from build123d import *

# Parameters (mm, degrees)
SKETCH1_W            = 20
SKETCH1_H            = 20
BOSS_EXTRUDE1_DEPTH  = 7.5
SKETCH1_3_W          = 20
SKETCH1_3_H          = 20
CUT_EXTRUDE2_DEPTH   = 1.5
SKETCH3_W            = 10
SKETCH3_H            = 20
BOSS_EXTRUDE2_DEPTH  = 1.5
MOUNTHOLE_DEPTH      = 17.007810594
MOUNTHOLE_DEPTH_BACK = 17.007810594
SKETCH5_R            = 1.5
SKETCH6_R            = 3.5
BEARINGHOLE_DEPTH    = 2.5
SKETCH4_R            = 2
SHAFT_DEPTH          = 5


with BuildPart() as part:
    # Sketch1 → Boss-Extrude1 (new, symmetric)
    with BuildSketch(Plane(origin=(0, 0, 0), x_dir=(1, 0, 0), z_dir=(0, 1, 0))):
        Rectangle(SKETCH1_W, SKETCH1_H)
    extrude(amount=BOSS_EXTRUDE1_DEPTH, both=True)

    # Sketch1_3 → Cut-Extrude2 (cut, symmetric)
    with BuildSketch(Plane(origin=(0, 0, 0), x_dir=(1, 0, 0), z_dir=(0, 1, 0))):
        Rectangle(SKETCH1_3_W, SKETCH1_3_H)
    extrude(amount=CUT_EXTRUDE2_DEPTH, both=True, mode=Mode.SUBTRACT)


with BuildPart() as cut_extrude2_piece_1:
    # of the separate pieces the step leaves, piece 1, a body of its own (cut_extrude2_pieces)
    add(part.part.solids().sort_by_distance((-10, -7.5, -10))[0])



with BuildPart() as cut_extrude2_piece_2:
    # of the separate pieces the step leaves, piece 2, a body of its own (cut_extrude2_pieces)
    add(part.part.solids().sort_by_distance((-10, 1.5, -10))[0])


with BuildPart() as cut_extrude2_piece_1_1:
    add(cut_extrude2_piece_1.part)

    add(cut_extrude2_piece_2.part)  # Boss-Extrude2 merges Cut-Extrude2 piece 2
    # Sketch3 → Boss-Extrude2 (add, symmetric)
    with BuildSketch(Plane(origin=(0, 0, 0), x_dir=(1, 0, 0), z_dir=(0, 1, 0))):
        with Locations((5, 0)):
            Rectangle(SKETCH3_W, SKETCH3_H)
    extrude(amount=BOSS_EXTRUDE2_DEPTH, both=True)

    # Sketch5 → mounthole (cut, two sides: drawn at the far end of the back side and taken through both)
    with BuildSketch(Plane(origin=(0, 0, 0), x_dir=(1, 0, 0), z_dir=(0, 1, 0)).offset(-MOUNTHOLE_DEPTH_BACK)):
        with Locations(Location((-5, 6, 0), (0, 0, 270))):
            Circle(SKETCH5_R)
        with Locations(Location((5, 6, 0), (0, 0, 270))):
            Circle(SKETCH5_R)
        with Locations(Location((5, -6, 0), (0, 0, 270))):
            Circle(SKETCH5_R)
        with Locations(Location((-5, -6, 0), (0, 0, 270))):
            Circle(SKETCH5_R)
    extrude(amount=MOUNTHOLE_DEPTH + MOUNTHOLE_DEPTH_BACK, mode=Mode.SUBTRACT)

    # Sketch6 → bearinghole (cut)
    with BuildSketch(Plane(origin=(5, 0, 0), x_dir=(0, 0, -1), z_dir=(1, 0, 0))):
        Circle(SKETCH6_R)
    extrude(amount=BEARINGHOLE_DEPTH, mode=Mode.SUBTRACT)

    # Sketch4 → shaft (cut)
    with BuildSketch(Plane(origin=(10, 0, 0), x_dir=(0, 0, -1), z_dir=(1, 0, 0))):
        Circle(SKETCH4_R)
    extrude(amount=-SHAFT_DEPTH, mode=Mode.SUBTRACT)


solid = cut_extrude2_piece_1_1.part
Work out the finished part from the listing and answer in its coordinate system (mm). A direction names the side the tool comes from. Give positions to 0.01 mm unless a question says otherwise; leave off trailing zeros. Order: outer loops, then holes, each group sorted by start corner. A loop starts at its lowest first (then second) coordinate and runs counter-clockwise, first axis right, second up. Notation, with made-up numbers: (46.5, 9) -> (56.5, 9) arc R23 ccw to (56.5, 29) -> close; hole circle Ø10 at (89, 70.25). An arc over 180 degrees is marked (long way). Answer as a JSON object with one key per item and string values. Group by question number.
1. The mould has two halves that part along Y. Classify faces 1 (the flat face through (-5, -1.5, 0)), 2 (the flat face through (7.5, -2, -2)), 3 (the flat face through (-10, -4, 0)), 4 (the flat face through (0, 7.5, 0)): released by +Y, released by -Y, zero draft, split by the parting line, or undercut.
2. Section A-A on x = -3 is taken. Determine the outline of the cut face in (y, z).
3. Section C-C on z = 6 is taken. Determine the outline of the cut face in (x, y).
4. Consider line 1 along Z through (x, y) = (-5, 5.9); line 2 along X through (y, z) = (4, -6); line 3 along Y through (x, z) = (-6.5, 5.25). Determine where each line is inside the solid, lowest interval first. Write a range as [from, to].
5. A tool of negligible diameter and unlimited length cuts with its end or side. For faces 5 (the cylindrical face through (6.232, -1.341, -3.233)), 6 (the cylindrical face through (-3.99, 4.46, 4.89)), 7 (the flat face through (10, 0.1, 2.4)), 8 (the cylindrical face through (9, -2, 0)), 9 (the flat face through (0, 0, 0)), from which of +Z, -Z, +X, -X, +Y, -Y can it reach the whole face along a straight path? Write none if from no direction.
6. Section D-D on y = 5.5 is taken. Determine the outline of the cut face in (x, z), plus the area to 3 significant figures.
7. Section B-B on y = 0 is taken. Determine the outline of the cut face in (x, z), plus the area to 3 significant figures.
Result sheet:
{
 "1": {"face 1": "undercut", "face 2": "undercut", "face 3": "zero draft", "face 4": "released by +Y"},
 "2": {"outline": "(-7.5, -10) -> (-1.5, -10) -> (-1.5, 10) -> (-7.5, 10) -> close; (1.5, -10) -> (7.5, -10) -> (7.5, 10) -> (1.5, 10) -> close"},
 "3": {"outline": "(-10, -7.5) -> (-6.5, -7.5) -> (-6.5, -1.5) -> (-10, -1.5) -> close; (-10, 1.5) -> (-6.5, 1.5) -> (-6.5, 7.5) -> (-10, 7.5) -> close; (-3.5, -7.5) -> (3.5, -7.5) -> (3.5, 7.5) -> (-3.5, 7.5) -> (-3.5, 1.5) -> (0, 1.5) -> (0, -1.5) -> (-3.5, -1.5) -> close; (6.5, -7.5) -> (10, -7.5) -> (10, 7.5) -> (6.5, 7.5) -> close"},
 "4": {"line 1": "z = [-10, -7.5], [-4.5, 4.5], [7.5, 10]", "line 2": "x = [-10, -6.5], [-3.5, 3.5], [6.5, 10]", "line 3": "y = [-7.5, -1.5], [1.5, 7.5]"},
 "5": {"face 5": "none", "face 6": "+Y, -Y", "face 7": "+Z, -Z, +X, +Y, -Y", "face 8": "+X", "face 9": "+Z, -Z, -X"},
 "6": {"outline": "(-10, -10) -> (10, -10) -> (10, 10) -> (-10, 10) -> close; hole circle Ø3 at (-5, -6); hole circle Ø3 at (-5, 6); hole circle Ø3 at (5, -6); hole circle Ø3 at (5, 6)", "area": "372 mm^2"},
 "7": {"outline": "(0, -10) -> (10, -10) -> (10, -2) -> (7.5, -2) -> (7.5, -3.5) -> (5, -3.5) -> (5, 3.5) -> (7.5, 3.5) -> (7.5, 2) -> (10, 2) -> (10, 10) -> (0, 10) -> close; hole circle Ø3 at (5, -6); hole circle Ø3 at (5, 6)", "area": "158 mm^2"}
}
